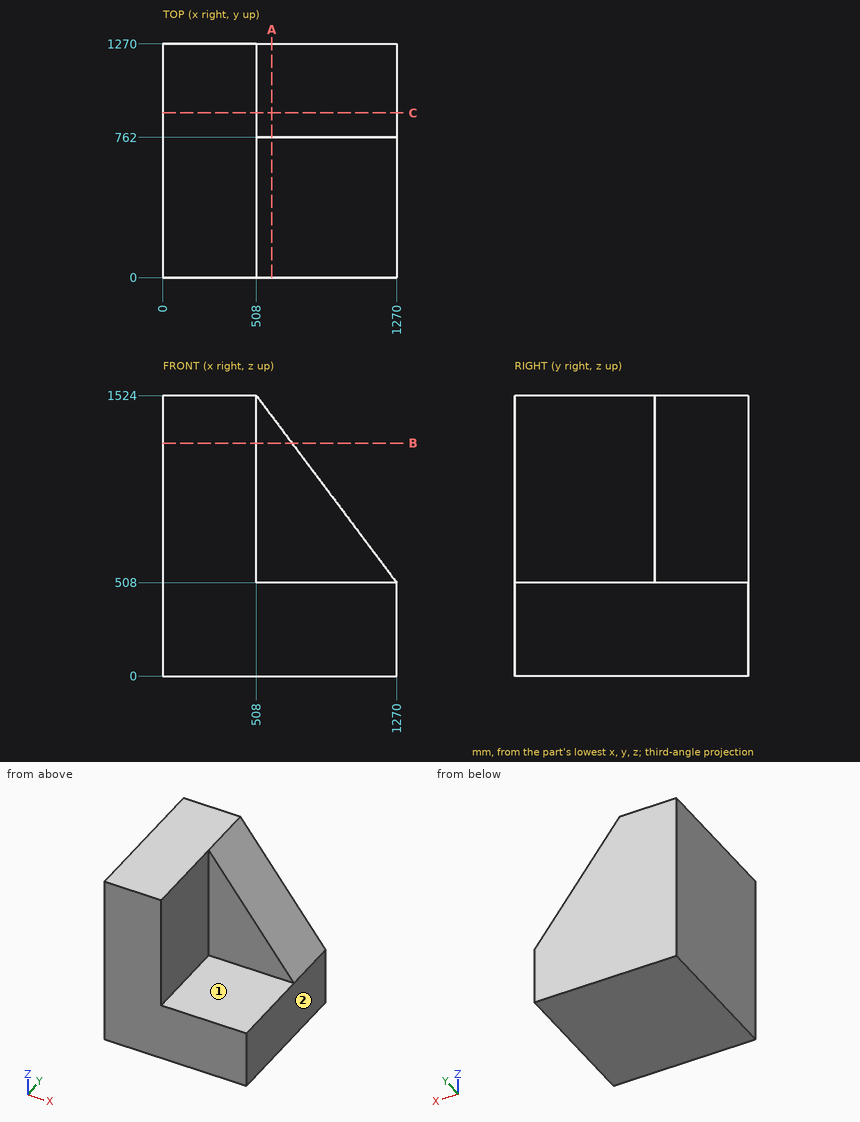
Could you check a few things on this drawing? It's one solid part, dimensions in mm from its lowest x, y, z. A direction names the side the tool comes from. Round coordinates to 2 decimals unless told otherwise and drop trailing zeros. Order: outer loops, then holes, each group sorted by start corner. A loop starts at its lowest first (then second) coordinate and runs counter-clockwise, first axis right, second up. Notation, with made-up numbers: M 25.5,11 L 52.5,11 A22 ccw 52.5,36 Z; hole C 63,58 d10. An arc over 180 degrees is marked long. One line per item, written item: value.
(1) Imagine slicing it at C-C (y = 895). Write out the boundary of the cut face in (x, z), and give its area (3 significant figures).
Ans:
outline: M 0,0 L 1270,0 L 1270,508 L 508,1524 L 0,1524 Z
area: 1,550,000 mm^2
(2) Imagine slicing it at A-A (x = 592). Write out the boundary of the cut face in (y, z).
Ans:
outline: M 0,0 L 1270,0 L 1270,1412 L 762,1412 L 762,508 L 0,508 Z
(3) Which directions (+Z, -Z, +X, -X, +Y, -Y) give clear straight access to the entire face, cutting with the end or side of a thin tool? Please do the marked faces 1 and 2.
Ans:
face 1: +Z, +X, -Y
face 2: +Z, -Z, +X, +Y, -Y
(4) Imagine slicing it at B-B (z = 1266). Write out the boundary of the cut face in (x, y), and give its area (3 significant figures).
Ans:
outline: M 0,0 L 508,0 L 508,762 L 701.5,762 L 701.5,1270 L 0,1270 Z
area: 743,000 mm^2
(5) I need wall thicknesses on line 1 along Y through (x, z) = (539, 1119.5); line 2 along Z through (x, y) = (561, 54.5). Which ranges of each line are inside material? Lowest first, please. Write a range as from..to.
Ans:
line 1: y = 762..1270
line 2: z = 0..508
(6) I'm going to push flat-ended pins straight in: P1, Ø5, axis at y = 729.5, z = 821, coming from the +X side; P2, Ø10, axis at x = 517.5, y = 730, coming from the +Z side. Where does each tip first touch, or does it pass through?
Ans:
P1: stops at x = 508
P2: stops at z = 508
